from build123d import *

# Parameters (mm, degrees)
CROQUIS2_W              = 120
CROQUIS2_H              = 120
SALIENTE_EXTRUIR2_DEPTH = 2.7
CROQUIS3_R              = 3
CORTAR_EXTRUIR1_DEPTH   = 85.895759611
CROQUIS4_W              = 13
CROQUIS4_H              = 5
CORTAR_EXTRUIR2_DEPTH   = 2.7


with BuildPart() as part:
    # Croquis2 → Saliente-Extruir2 (new body)
    with BuildSketch(Plane(origin=(0, 0, 0), x_dir=(1, 0, 0), z_dir=(0, 1, 0))):
        Rectangle(CROQUIS2_W, CROQUIS2_H)
    extrude(amount=SALIENTE_EXTRUIR2_DEPTH)

    # Croquis3 → Cortar-Extruir1 (cut, through all)
    with BuildSketch(Plane(origin=(0, 2.7, 0), x_dir=(1, 0, 0), z_dir=(0, 1, 0))):
        with Locations(Location((0, 50, 0), (0, 0, 270))):
            Circle(CROQUIS3_R)
        with Locations(Location((40, 50, 0), (0, 0, 270))):
            Circle(CROQUIS3_R)
        with Locations(Location((-40, 50, 0), (0, 0, 270))):
            Circle(CROQUIS3_R)
        with Locations(Location((-40, -50, 0), (0, 0, 270))):
            Circle(CROQUIS3_R)
        with Locations(Location((40, -50, 0), (0, 0, 270))):
            Circle(CROQUIS3_R)
        with Locations(Location((0, -50, 0), (0, 0, 270))):
            Circle(CROQUIS3_R)
    extrude(amount=-CORTAR_EXTRUIR1_DEPTH, mode=Mode.SUBTRACT)

    # Croquis4 → Cortar-Extruir2 (cut)
    with BuildSketch(Plane.XZ):
        with Locations((-27.5, -31.5)):
            Rectangle(CROQUIS4_W, CROQUIS4_H)
    extrude(amount=-CORTAR_EXTRUIR2_DEPTH, mode=Mode.SUBTRACT)


solid = part.part
Model file for the job. Use its own axes, mm. A direction names the side the tool comes from. Give positions to 0.01 mm unless a question says otherwise; leave off trailing zeros. Loops run counter-clockwise (first coordinate to the right, second up) from the corner with the lowest first, then second, coordinate; pieces in that order, holes last.
1) Saw through at A-A (z = -50). Write the cut outline in (x, y).
2) Tool access for faces 1 (the flat face through (-1, 1, -60)), 2 (the flat face through (-21, 1, -32)): list every direction of +Z, -Z, +X, -X, +Y, -Y with a clear straight run to the whole face (end or side of a thin tool).
3) Pull direction X, two halves, no side cores. Call faces 3 (the cylindrical face through (42.03, 1.37, -52.21)), 4 (the flat face through (-1, 1, 60)), 5 (the flat face through (-60, 1, 1)), 6 (the cylindrical face through (0, 1, 47)): +X half, -X half, draft (parallel to the pull), parting line (faces both ways), or undercut.
4) Saw through at B-B (x = -40). Write the cut outline in (y, z), plus the area to 3 significant figures.
5) Flat gauge pin, fed straight in: pin 1 Ø9.5 at (x, z) = (-40, -50) entering from +Y. Where does the tip first touch, or does it go through?
6) Wall check: line 1 (X direction, y = 1.1, z = 50); line 2 (Z direction, x = -31, y = 1.55). Give the ranges that are in metal, low to high.
7) Saw through at C-C (y = 1). Write the cut outline in (x, z).
Answer block:
1. outline: (-60, 0) - (-43, 0) - (-43, 2.7) - (-60, 2.7) - close; (-37, 0) - (-3, 0) - (-3, 2.7) - (-37, 2.7) - close; (3, 0) - (37, 0) - (37, 2.7) - (3, 2.7) - close; (43, 0) - (60, 0) - (60, 2.7) - (43, 2.7) - close
2. face 1: -Z, +X, -X, +Y, -Y
2. face 2: +Y, -Y
3. face 3: undercut
3. face 4: draft
3. face 5: -X half
3. face 6: undercut
4. outline: (0, -60) - (2.7, -60) - (2.7, -53) - (0, -53) - close; (0, -47) - (2.7, -47) - (2.7, 47) - (0, 47) - close; (0, 53) - (2.7, 53) - (2.7, 60) - (0, 60) - close
4. area: 292 mm2
5. pin 1: stops at y = 2.7
6. line 1: x = -60 to -43, -37 to -3, 3 to 37, 43 to 60
6. line 2: z = -60 to -34, -29 to 60
7. outline: (-60, -60) - (60, -60) - (60, 60) - (-60, 60) - close; hole circle Ø6 at (-40, -50); hole circle Ø6 at (-40, 50); hole (-34, -34) - (-21, -34) - (-21, -29) - (-34, -29) - close; hole circle Ø6 at (0, -50); hole circle Ø6 at (0, 50); hole circle Ø6 at (40, -50); hole circle Ø6 at (40, 50)
